Drawing for the job (mm, zero at the part's lowest x, y, z). A direction names the side the tool comes from. Give positions to 0.01 mm unless a question says otherwise; leave off trailing zeros. Write each loop counter-clockwise with the first axis right and the second up, starting at its lowest first coordinate (ties: lowest second). Pieces come first, ordered by that corner, then holes. Notation, with made-up numbers: M 8,45 L 27,45 A27 ccw 27,83 Z; hole C 24,2.5 d5. An arc over 180 degrees is marked long. Answer as a JSON object with one key per item and string values. Group by question number.
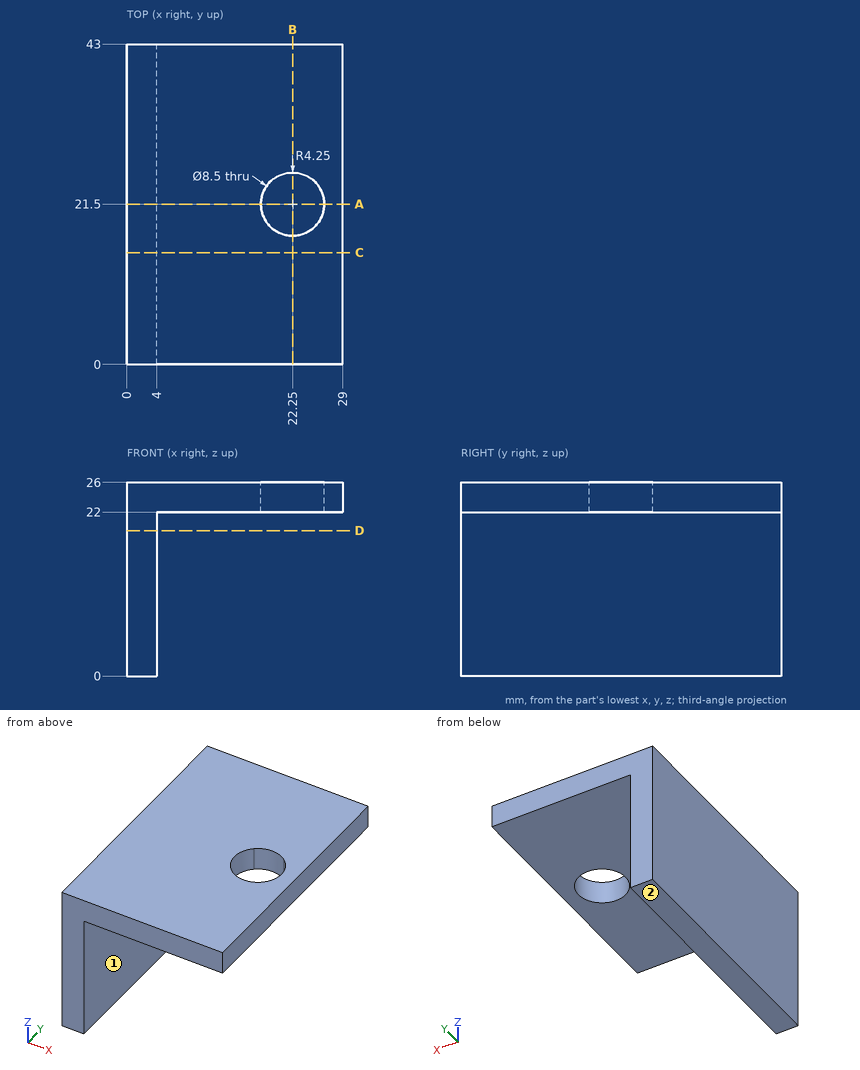
Q1. Slice it at A-A, the plane y = 21.5. Write the cut outline in (x, z), then the cut area to 3 significant figures.
Q2. Drop flat-ended pins along their axis: P1, Ø1.5, axis at x = 6, z = 20, coming from the -Y side; P2, Ø2, axis at y = 19, z = 17.5, coming from the +X side; P3, Ø12.5, axis at x = 18.5, y = 14, coming from the -Z side. Give the stop position or say it passes through.
Q3. Slice it at C-C, the plane y = 15. Write the cut outline in (x, z).
Q4. Slice it at B-B, the plane x = 22.25. Write the cut outline in (y, z).
Q5. Slice it at D-D, the plane z = 19.5. Write the cut outline in (x, y).
Q6. 3-axis set-ups, long thin cutter, end or side, ignore diameter. For the marked faces 1 and 2: which of +Z, -Z, +X, -X, +Y, -Y reach the whole face in a straight line?
Q7. Wall check: L1, parallel to Y at x = 22.25, z = 23.4; L2, parallel to X at y = 21.5, z = 24.45; L3, parallel to X at y = 24.5, z = 1.75. Give the ranges that are in metal, low to high.
Solved:
{
 "1": {"outline": "M 0,0 L 4,0 L 4,22 L 18,22 L 18,26 L 0,26 Z; M 26.5,22 L 29,22 L 29,26 L 26.5,26 Z", "area": "170 mm²"},
 "2": {"P1": "passes through", "P2": "stops at x = 4", "P3": "stops at z = 22"},
 "3": {"outline": "M 0,0 L 4,0 L 4,22 L 29,22 L 29,26 L 0,26 Z"},
 "4": {"outline": "M 0,22 L 17.25,22 L 17.25,26 L 0,26 Z; M 25.75,22 L 43,22 L 43,26 L 25.75,26 Z"},
 "5": {"outline": "M 0,0 L 4,0 L 4,43 L 0,43 Z"},
 "6": {"face 1": "-Z, +X, +Y, -Y", "face 2": "-Z, +X, -X, +Y, -Y"},
 "7": {"L1": "y = 0 to 17.25, 25.75 to 43", "L2": "x = 0 to 18, 26.5 to 29", "L3": "x = 0 to 4"}
}
